from build123d import *

# Parameters (mm, degrees)
BASEHEAD_DEPTH      = 7.76
SKETCH4_W           = 0.6
SKETCH4_H           = 11.392304845
BOSS_EXTRUDE1_DEPTH = 10


# Read off the part's stored shape, not the designer's step: HeadChamfer
with BuildPart() as part:
    # Sketch1 → BaseHead (new body)
    with BuildSketch(Plane(origin=(0, 0, 0), x_dir=(0, 0, -1), z_dir=(1, 0, 0))):
        Polygon((9, 5.196152423), (9, -5.196152423), (0, -10.392304845), (-9, -5.196152423), (-9, 5.196152423), (0, 10.392304845), align=None)
    extrude(amount=BASEHEAD_DEPTH)

    # HeadChamfer outline → HeadChamfer (revolve, cut)
    with BuildSketch(Plane.YX):
        Polygon((10.392304847, 0.803847578), (9, 0), (10.392304847, 0), align=None)
    revolve(axis=Axis((0, 0, 0), (1, 0, 0)), mode=Mode.SUBTRACT)

    # HeadChamfer 2 outline → HeadChamfer 2 (revolve)
    with BuildSketch(Plane.YX):
        Polygon((6, 7.76), (6, 46.796), (5.036, 47.76), (0, 47.76), (0, 7.76), align=None)
    revolve(axis=Axis((0, 0, 0), (1, 0, 0)))

    # Sketch4 → BearingFace (revolve, cut)
    with BuildSketch(Plane.XY, mode=Mode.PRIVATE) as bearingface_sk:
        with Locations((7.46, 14.696152423)):
            Rectangle(SKETCH4_W, SKETCH4_H)
    revolve(bearingface_sk.sketch.rotate(Axis((0, 0, 0), (1, 0, 0)), 90), axis=Axis((0, 0, 0), (1, 0, 0)), mode=Mode.SUBTRACT)

    # Sketch5 → Boss-Extrude1 (add)
    with BuildSketch(Plane(origin=(42.76, 0, 0), x_dir=(0, 0, -1), z_dir=(1, 0, 0))):
        Polygon((0, 10.392304845), (-9, 5.196152423), (-9, -5.196152423), (0, -10.392304845), (9, -5.196152423), (9, 5.196152423), align=None)
    extrude(amount=-BOSS_EXTRUDE1_DEPTH)


solid = part.part
Geometry check sheet. Reference: the model listing, model coordinates, mm. A direction names the side the tool comes from. Give positions to 0.01 mm unless a question says otherwise; leave off trailing zeros. Order: outer loops, then holes, each group sorted by start corner. A loop starts at its lowest first (then second) coordinate and runs counter-clockwise, first axis right, second up. Notation, with made-up numbers: (-0.75, 6.25) - (3.25, 6.25) arc R13 cw to (3.25, 30.25) - close; hole circle Ø11 at (66.25, 52). An arc over 180 degrees is marked (long way). Answer as a JSON object with one key per item and string values.
(1) Material ranges on line 1 (X direction, y = 7, z = 3); line 2 (Y direction, x = 23, z = -3.25), recorded low to high.
Report:
{"line 1": "0 to 7.76, 32.76 to 42.76", "line 2": "-5.04 to 5.04"}
(2) Tool access check on faces 4 (the cylindrical face through (20, -6, 0)), 5 (the flat face through (7.16, -4.5, 8.1)), 6 (the flat face through (7.16, -4.5, -8.1)). Record the directions out of +Z, -Z, +X, -X, +Y, -Y that give a thin tool (end or side, any length) a straight path to the whole face; none if there is none.
Report:
{"face 4": "none", "face 5": "+Z, -Y", "face 6": "-Z, -Y"}
(3) Cross-section at A-A (x = 33.5). Record the cut outline in (y, z).
Report:
{"outline": "(-10.39, 0) - (-5.2, -9) - (5.2, -9) - (10.39, 0) - (5.2, 9) - (-5.2, 9) - close"}
(4) Draft check along X on faces 1 (the flat face through (7.16, 9.3, 0)), 2 (the flat face through (38, 0, 9)), 3 (the conical face through (0.192, -4.686, -8.07)). Enter one of: released by +X, released by -X, zero draft, split by the parting line, or undercut.
Report:
{"face 1": "undercut", "face 2": "zero draft", "face 3": "released by -X"}
(5) Cross-section at B-B (x = 43.5). Record the cut outline in (y, z), then the cut area to 3 significant figures.
Report:
{"outline": "circle Ø12 at (0, 0)", "area": "113 mm^2"}
(6) Depth check by flat-ended pin: pin 1 Ø5 at (y, z) = (-3, -7) entering from +X; pin 2 Ø1.5 at (x, y) = (25, -5) entering from -Z; pin 3 Ø1.5 at (y, z) = (8, 2.5) entering from -X; pin 4 Ø3 at (y, z) = (-9, 0.5) entering from +X. Enter the tip coordinate at first touch or a pass-through.
Report:
{"pin 1": "x = 47.68", "pin 2": "z = -4.24", "pin 3": "x = 0", "pin 4": "x = 42.76"}
